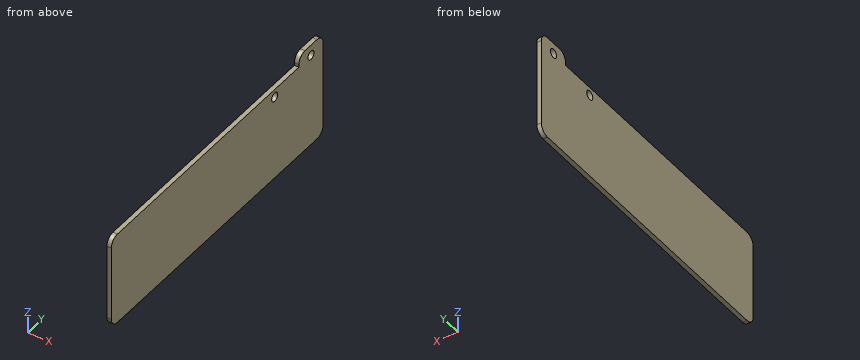
from build123d import *

# Parameters (mm, degrees)
F0_R     = 5
F1_DEPTH = 5


with BuildPart() as f1:
    # F0 (on Right) → F1 (new body)
    with BuildSketch(Plane.YZ):
        with BuildLine():
            Line((-20, -1), (-320, -1))
            ThreePointArc((-320, -1), (-327.071068, -3.928932), (-330, -11))
            Line((-330, -11), (-330, -95))
            ThreePointArc((-330, -95), (-327.071068, -102.071068), (-320, -105))
            Line((-320, -105), (10, -105))
            ThreePointArc((10, -105), (17.071068, -102.071068), (20, -95))
            Line((20, -95), (20, 2))
            ThreePointArc((20, 2), (17.071068, 9.071068), (10, 12))
            Line((10, 12), (-10, 12))
            ThreePointArc((-10, 12), (-17.071068, 9.071068), (-20, 2))
            Line((-20, 2), (-20, -1))
        make_face()
        with Locations((-60, -10)):
            Circle(F0_R, mode=Mode.SUBTRACT)
        Circle(F0_R, mode=Mode.SUBTRACT)
    extrude(amount=F1_DEPTH)


solid = f1.part
Work out the finished part from the listing and answer in its coordinate system (mm). Round coordinates to 2 decimals unless told otherwise and drop trailing zeros. Write each loop counter-clockwise with the first axis right and the second up, starting at its lowest first coordinate (ties: lowest second). Pieces come first, ordered by that corner, then holes. Notation, with made-up numbers: (77, 21) -> (87, 21) arc R31 cw to (87, 55) -> close; hole circle Ø10 at (88, 12.5). An arc over 180 degrees is marked (long way). Answer as CSV lines item,"result". Start each with the question number.
(1) The part is cut by section A-A, the plane y = 0. Give the vertices of the cut face in (x, z).
(2) The part is cut by section C-C, the plane y = -60. Give the vertices of the cut face in (x, z), then the cut area to 3 significant figures.
(3) The part is cut by section B-B, the plane x = 3.5. Give the vertices of the cut face in (y, z), then the cut area to 3 significant figures.
(4) Find the intervals of material crossed by probe 1 along Z at (x, y) = (1.1, 0); probe 2 along Z at (x, y) = (3.9, -60); probe 3 along Z at (x, y) = (1.9, -137), in increasing order.
(5) The part is cut by section D-D, the plane y = -287. Give the vertices of the cut face in (x, z).
(6) Each of these flat-tipped pins is pushed along its axis until it touches: pin 1 (2.5 mm diameter, centred on x = 1.5, y = -228, fed in from +Z); pin 2 (13 mm diameter, centred on y = -60, z = -10, fed in from +X); pin 3 (9 mm diameter, centred on y = 0, z = 0, fed in from -X). Where does it stop, or does it pass through?
Output values:
1,outline,"(0, -105) -> (5, -105) -> (5, -5) -> (0, -5) -> close; (0, 5) -> (5, 5) -> (5, 12) -> (0, 12) -> close"
2,outline,"(0, -105) -> (5, -105) -> (5, -15) -> (0, -15) -> close; (0, -5) -> (5, -5) -> (5, -1) -> (0, -1) -> close"
2,area,"470 mm²"
3,outline,"(-330, -95) arc R10 ccw to (-320, -105) -> (10, -105) arc R10 ccw to (20, -95) -> (20, 2) arc R10 ccw to (10, 12) -> (-10, 12) arc R10 ccw to (-20, 2) -> (-20, -1) -> (-320, -1) arc R10 ccw to (-330, -11) -> close; hole circle Ø10 at (-60, -10); hole circle Ø10 at (0, 0)"
3,area,"36,700 mm²"
4,probe 1,"z = -105 to -5, 5 to 12"
4,probe 2,"z = -105 to -15, -5 to -1"
4,probe 3,"z = -105 to -1"
5,outline,"(0, -105) -> (5, -105) -> (5, -1) -> (0, -1) -> close"
6,pin 1,"stops at z = -1"
6,pin 2,"stops at x = 5"
6,pin 3,"passes through"
